Work out the finished part from the listing and answer in its coordinate system (mm). A direction names the side the tool comes from. Give positions to 0.01 mm unless a question says otherwise; leave off trailing zeros. Order: outer loops, then holes, each group sorted by start corner. A loop starts at its lowest first (then second) coordinate and runs counter-clockwise, first axis right, second up. Notation, with made-up numbers: M 58.25,7.25 L 95.25,7.25 A28 ccw 95.25,36.25 Z; hole C 53.25,37 d8. An arc over 180 degrees is marked long. One line per item, written item: value.
from build123d import *

# Parameters (mm, degrees)
BOSS_EXTRUDE1_DEPTH = 4
SKETCH2_OUTSIDE_W   = 44.472
SKETCH2_OUTSIDE_H   = 42.46
SKETCH2_OUTSIDE_R   = 6.5
CUT_EXTRUDE2_DEPTH  = 11.704360482
CUT_EXTRUDE2_DRAFT  = -45
SKETCH3_R           = 4
BOSS_EXTRUDE2_DEPTH = 61


with BuildPart() as part:
    # Sketch1 → Boss-Extrude1 (new body)
    with BuildSketch(Plane(origin=(0, 0, 0), x_dir=(1, 0, 0), z_dir=(0, 1, 0))):
        Polygon((7.505553499, 0), (3.75277675, 6.5), (-3.75277675, 6.5), (-7.505553499, 0), (-3.75277675, -6.5), (3.75277675, -6.5), align=None)
    extrude(amount=BOSS_EXTRUDE1_DEPTH)


with BuildPart() as cut_extrude2_tool:
    # Sketch2 outside → Cut-Extrude2 (with draft: the straight prism first)
    with BuildSketch(Plane(origin=(0, 0, 0), x_dir=(-1, 0, 0), z_dir=(0, -1, 0))):
        Rectangle(SKETCH2_OUTSIDE_W, SKETCH2_OUTSIDE_H)
        Circle(SKETCH2_OUTSIDE_R, mode=Mode.SUBTRACT)
    extrude(amount=-CUT_EXTRUDE2_DEPTH)
    # Cut-Extrude2: the draft: its side faces are tilted about the plane it starts from
    cut_extrude2_sides = [cut_extrude2_tool.faces().sort_by_distance(p)[0] for p in [
        (0, 5.852180241, 21.23),
        (-22.236, 5.852180241, 0),
        (0, 5.852180241, -21.23),
        (22.236, 5.852180241, 0),
        (6.5, 5.852180241, 0),
    ]]
    draft(cut_extrude2_sides, Plane(origin=(0, 0, 0), x_dir=(-1, 0, 0), z_dir=(0, -1, 0)), CUT_EXTRUDE2_DRAFT)


with BuildPart() as part_1:
    add(part.part)

    # Cut-Extrude2: cut by cut_extrude2_tool
    add(cut_extrude2_tool.part, mode=Mode.SUBTRACT)

    # Sketch3 → Boss-Extrude2 (add)
    with BuildSketch(Plane(origin=(0, 4, 0), x_dir=(1, 0, 0), z_dir=(0, 1, 0))):
        with Locations(Location((0, 0, 0), (0, 0, 90))):
            Circle(SKETCH3_R)
    extrude(amount=BOSS_EXTRUDE2_DEPTH)


solid = part_1.part
(1) Which of the six approach directions +Z, -Z, +X, -X, +Y, -Y give full straight-line access (tool end or side, diameter ignored) to faces 1 (the conical face through (6.7, 0.2, 0)), 2 (the flat face through (3, 4, -3))?
Findings:
face 1: +X, -Y
face 2: +Y
(2) Section A-A, the plane y = 46 is taken. Give the vertices of the cut face in (x, z).
Findings:
outline: C 0,0 d8
(3) Given P1, Ø4, axis at x = 4.5, y = 36, coming from the -Z side; P2, Ø1.5, axis at x = 2, y = 7, coming from the -Z side; P3, Ø6, axis at x = 3, y = 23, coming from the -Z side; P4, Ø5, axis at x = -3.5, z = 0.5, coming from the -Y side, each flat-ended and moving along its own axis, determine where each tip first touches the part or whether it passes through.
Findings:
P1: stops at z = -3.12
P2: stops at z = -3.8
P3: stops at z = -4
P4: stops at y = 0
(4) Find the intervals of material crossed by probe 1 along Y at (x, z) = (4.5, 3.75); probe 2 along Z at (x, y) = (-0.75, 55); probe 3 along Z at (x, y) = (-2.5, 44), in increasing order. Write a range as from..to.
Findings:
probe 1: y = 0..4
probe 2: z = -3.93..3.93
probe 3: z = -3.12..3.12
